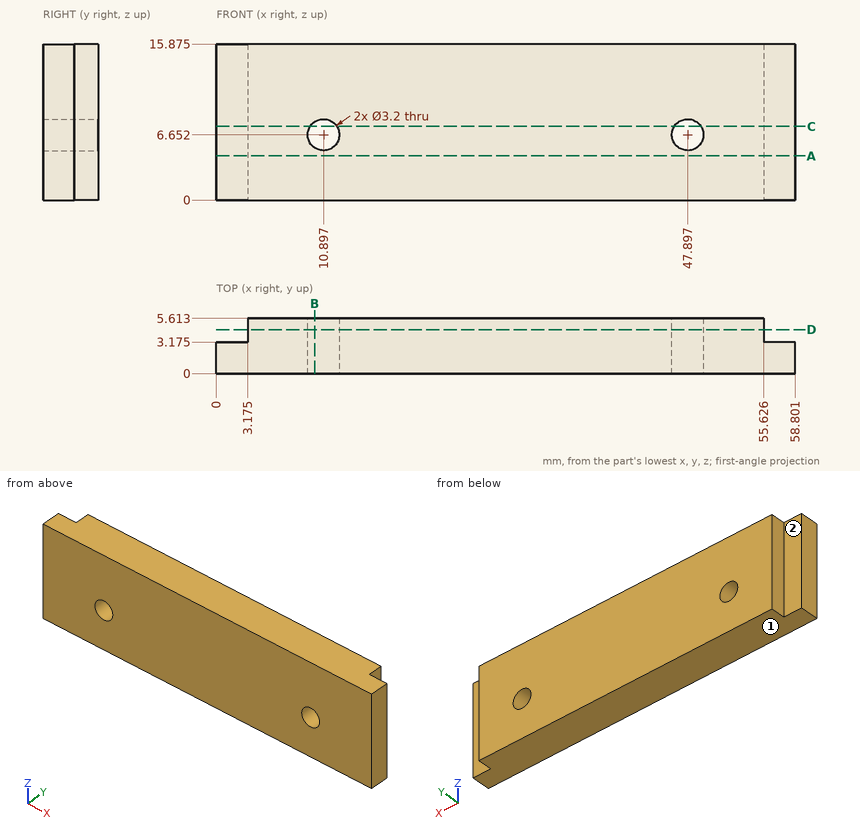
Part print with two shaded views. Sizes in mm from the minimum x, y, z corner. A direction names the side the tool comes from. Round coordinates to 2 decimals unless told otherwise and drop trailing zeros. Order: outer loops, then holes, each group sorted by start corner. A loop starts at its lowest first (then second) coordinate and runs counter-clockwise, first axis right, second up. Notation, with made-up numbers: (0.5, 16.25) -> (58.5, 16.25) arc R33 ccw to (58.5, 52.25) -> close; hole circle Ø1 at (85.25, 7). An arc over 180 degrees is marked (long way). One line per question, with ' | ' between items.
Q1. Slice it at C-C (z = 7.5). Write the cut outline in (x, y) (1 decimal), then the cut area to 3 significant figures.
Completed:
outline: (0, 0) -> (9.5, 0) -> (9.5, 5.6) -> (3.2, 5.6) -> (3.2, 3.2) -> (0, 3.2) -> close; (12.3, 0) -> (46.5, 0) -> (46.5, 5.6) -> (12.3, 5.6) -> close; (49.3, 0) -> (58.8, 0) -> (58.8, 3.2) -> (55.6, 3.2) -> (55.6, 5.6) -> (49.3, 5.6) -> close | area: 284 mm^2
Q2. Which spindle directions (+Z, -Z, +X, -X, +Y, -Y) get a long thin tool onto all of the face, cutting with end or side? Do the marked faces 1 and 2. Say none if no direction does.
Completed:
face 1: -Z, +X, -X, +Y, -Y | face 2: +Z, -Z, -X, +Y
Q3. Slice it at B-B (x = 10). Write the cut outline in (y, z) (1 decimal).
Completed:
outline: (0, 0) -> (5.6, 0) -> (5.6, 5.3) -> (0, 5.3) -> close; (0, 8) -> (5.6, 8) -> (5.6, 15.9) -> (0, 15.9) -> close
Q4. Drop flat-ended pins along their axis: pin 1 (0.7 mm diameter, centred on y = 4, z = 9, fed in from +X); pin 2 (3 mm diameter, centred on x = 10.9, z = 6.65, fed in from +Y); pin 3 (4 mm diameter, centred on x = 47.9, z = 6.65, fed in from +Y); pin 4 (1.6 mm diameter, centred on x = 57, z = 8, fed in from +Y) (3 decimals). Give the stop position or say it passes through.
Completed:
pin 1: stops at x = 55.63 | pin 2: passes through | pin 3: stops at y = 5.61 | pin 4: stops at y = 3.175
Q5. Slice it at A-A (z = 4.5). Write the cut outline in (x, y) (1 decimal).
Completed:
outline: (0, 0) -> (58.8, 0) -> (58.8, 3.2) -> (55.6, 3.2) -> (55.6, 5.6) -> (3.2, 5.6) -> (3.2, 3.2) -> (0, 3.2) -> close
Q6. Probe probe 1 along X at (y, z) = (2.7, 8) (1 decimal); probe 2 along X at (y, z) = (3.7, 6) (1 decimal); probe 3 along X at (y, z) = (3.6, 1.25) (1 decimal). List the from-to ranges inside material, lowest first.
Completed:
probe 1: x = 0 to 10, 11.8 to 47, 48.8 to 58.8 | probe 2: x = 3.2 to 9.4, 12.4 to 46.4, 49.4 to 55.6 | probe 3: x = 3.2 to 55.6
Q7. Slice it at D-D (y = 4.45). Write the cut outline in (x, z) (1 decimal).
Completed:
outline: (3.2, 0) -> (55.6, 0) -> (55.6, 15.9) -> (3.2, 15.9) -> close; hole circle Ø3.2 at (10.9, 6.7); hole circle Ø3.2 at (47.9, 6.7)
